Geometry: final body of the model. Coordinates: model frame, mm. Round coordinates to 2 decimals unless told otherwise and drop trailing zeros. Loops run counter-clockwise (first coordinate to the right, second up) from the corner with the lowest first, then second, coordinate; pieces in that order, holes last. Notation, with made-up numbers: M 72,72.5 L 131,72.5 A13 cw 131,92.5 Z; hole C -38,56.25 d10. An arc over 180 degrees is marked long. Return JSON: item names as keys, results as strings.
Autodesk Inventor part; units mm, degrees
ref_plane "YZ Plane" through (0, 0, 0) normal (1, 0, 0) x (0, 1, 0)
ref_plane "XZ Plane" through (0, 0, 0) normal (0, 1, 0) x (-1, 0, 0)
ref_plane "XY Plane" through (0, 0, 0) normal (0, 0, 1) x (1, 0, 0)
sketch "Skizze1" plane through (0, 0, 0) normal (0, 0, 1) x (1, 0, 0)
  line L0 (-45, -37) -> (45, -37)
  line L1 (45, -37) -> (45, 43)
  line L2 (45, 43) -> (-45, 43)
  line L3 (-45, 43) -> (-45, -37)
  line L4 (0, 59) -> (0, -53)
  point P0 (0, 0)
  dimension "d0" = 90
  dimension "d2" = 37
  dimension "d14" = 80
extrude "Extrusion1" add sketch "Skizze1" along normal blind 1.6
sketch "Skizze2" plane through (0, 0, 1.6) normal (0, 0, 1) x (1, 0, 0)
  line L0 (-45, -37) -> (45, -37)
  line L1 (45, -37) -> (45, 43)
  line L2 (45, 43) -> (-45, 43)
  line L3 (-45, 43) -> (-45, -37)
  line L4 (-42, -34) -> (42, -34)
  line L5 (42, -34) -> (42, 40)
  line L6 (42, 40) -> (-42, 40)
  line L7 (-42, 40) -> (-42, -34)
  line L8 (0, 59) -> (0, -53)
  point P0 (0, 0)
  point P1 (42, -34)
  dimension "d5" = 3
hole "Montage" at (-42, 40, 1.6) at (42, 40, 1.6) at (42, -34, 1.6) at (-42, -34, 1.6) direction (0, 0, -1) diameter 3 end through all
sketch "Skizze3" plane through (0, 0, 1.6) normal (0, 0, 1) x (1, 0, 0)
  line L0 (29, -34) -> (36, -34) construction
  circle A0 centre (42, 40) radius 1.5
  circle A1 centre (-42, 40) radius 1.5
  circle A2 centre (42, -34) radius 1.5
  line L1 (-45, -37) -> (45, -37)
  line L2 (45, -37) -> (45, 43)
  line L3 (45, 43) -> (-45, 43)
  line L4 (-45, 43) -> (-45, -37)
  point P0 (0, 0)
  dimension "d27" = 7
  dimension "d29" = 3
  dimension "d30" = 9
hole "Akku" at (36, -34, 1.6) at (29, -34, 1.6) direction (0, 0, -1) diameter 4 end through all
sketch "Skizze4" plane through (0, 0, 1.6) normal (0, 0, 1) x (1, 0, 0)
  circle A0 centre (29, -34) radius 2
sketch "Skizze5" plane through (0, 0, 1.6) normal (0, 0, 1) x (1, 0, 0)
  circle A0 centre (36, -34) radius 2
fillet "Rundung3" radius 2 4 edges at (45, -37, 0.8) (45, 43, 0.8) (-45, 43, 0.8) (-45, -37, 0.8)
properties part number "Powerboard" material "Phenolharz"
Q1. Material intervals for L1, parallel to Y at x = -42, z = 0.85; L2, parallel to X at y = -34, z = 0.6; L3, parallel to X at y = 40, z = 1.2, sorted ascending.
Determined:
{"L1": "y = -37 to -35.5, -32.5 to 38.5, 41.5 to 43", "L2": "x = -45 to -43.5, -40.5 to 27, 31 to 34, 38 to 40.5, 43.5 to 45", "L3": "x = -45 to -43.5, -40.5 to 40.5, 43.5 to 45"}
Q2. Section query D-D (x = 36). Output: boundary loops of the cut face in (y, z).
Determined:
{"outline": "M -37,0 L -36,0 L -36,1.6 L -37,1.6 Z; M -32,0 L 43,0 L 43,1.6 L -32,1.6 Z"}
Q3. Pull-direction query (X, two-part tool) for faces 1 (the cylindrical face through (37.774, -34.923, 0.789)), 2 (the flat face through (-1, 4, 1.6)), 3 (the cylindrical face through (-44.4, 42.43, 0.81)); classes: pulls with the +X half, pulls with the -X half, needs draft (parallel to the pull), parting line crosses it, or undercut.
Determined:
{"face 1": "undercut", "face 2": "needs draft", "face 3": "pulls with the -X half"}
Q4. Section query B-B (y = 40). Output: boundary loops of the cut face in (x, z), plus the area to 3 significant figures.
Determined:
{"outline": "M -45,0 L -43.5,0 L -43.5,1.6 L -45,1.6 Z; M -40.5,0 L 40.5,0 L 40.5,1.6 L -40.5,1.6 Z; M 43.5,0 L 45,0 L 45,1.6 L 43.5,1.6 Z", "area": "134 mm^2"}
Q5. Section query A-A (y = -34). Output: boundary loops of the cut face in (x, z), plus the area to 3 significant figures.
Determined:
{"outline": "M -45,0 L -43.5,0 L -43.5,1.6 L -45,1.6 Z; M -40.5,0 L 27,0 L 27,1.6 L -40.5,1.6 Z; M 31,0 L 34,0 L 34,1.6 L 31,1.6 Z; M 38,0 L 40.5,0 L 40.5,1.6 L 38,1.6 Z; M 43.5,0 L 45,0 L 45,1.6 L 43.5,1.6 Z", "area": "122 mm^2"}
Q6. Section query C-C (x = -42). Output: boundary loops of the cut face in (y, z), plus the area to 3 significant figures.
Determined:
{"outline": "M -37,0 L -35.5,0 L -35.5,1.6 L -37,1.6 Z; M -32.5,0 L 38.5,0 L 38.5,1.6 L -32.5,1.6 Z; M 41.5,0 L 43,0 L 43,1.6 L 41.5,1.6 Z", "area": "118 mm^2"}
